```python
from build123d import *

# Parameters (mm, degrees)
EXTRUDE_1_DEPTH     = 30
SKETCH_2_R          = 10
CUT_EXTRUDE_1_DEPTH = 15
EXTRUDE_START       = 20
SKETCH_3_R          = 12.5
SKETCH_3_R_2        = 10
EXTRUDE_2_DEPTH     = 20


with BuildPart() as part:
    # 草图1 → 凸台-拉伸1 (new body)
    with BuildSketch(Plane(origin=(0, 0, 0), x_dir=(0, 0, -1), z_dir=(1, 0, 0))):
        Polygon((-1000, 30), (1000, 30), (1000, 0), (15, 0), (15, 15), (-15, 15), (-15, 0), (-1000, 0), align=None)
    extrude(amount=EXTRUDE_1_DEPTH)

    # 草图2 → 切除-拉伸1 (cut)
    with BuildSketch(Plane.XZ):
        with Locations(Location((15, 883.8834765, 0), (0, 0, 270))):
            Circle(SKETCH_2_R)
        with Locations(Location((15, -883.8834765, 0), (0, 0, 90))):
            Circle(SKETCH_2_R)
    extrude(amount=-CUT_EXTRUDE_1_DEPTH, mode=Mode.SUBTRACT)

    # 草图3 → 凸台-拉伸2 (add)
    # profile 1 of 2: a face of its own
    with BuildSketch(Plane.XZ.offset(EXTRUDE_START)):
        with Locations(Location((15, 883.8834765, 0), (0, 0, 90))):
            Circle(SKETCH_3_R)
        with Locations(Location((15, 883.8834765, 0), (0, 0, 270))):
            Circle(SKETCH_3_R_2, mode=Mode.SUBTRACT)
    # profile 2 of 2: a face of its own
    with BuildSketch(Plane.XZ.offset(EXTRUDE_START)):
        with Locations(Location((15, -883.8834765, 0), (0, 0, 90))):
            Circle(SKETCH_3_R)
        with Locations(Location((15, -883.8834765, 0), (0, 0, 90))):
            Circle(SKETCH_3_R_2, mode=Mode.SUBTRACT)
    extrude(amount=-EXTRUDE_2_DEPTH)


solid = part.part
```
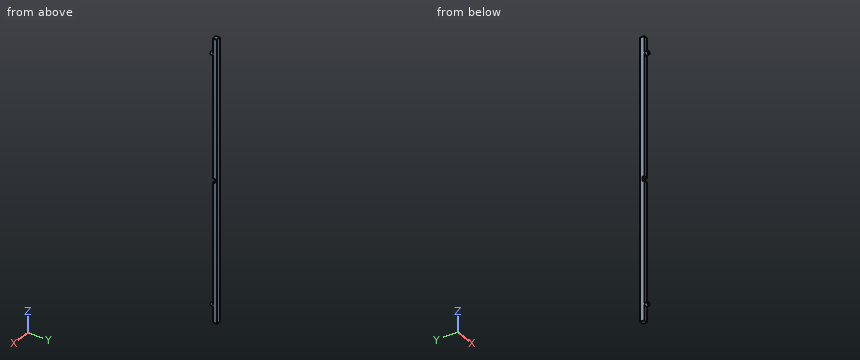
Input: part model. Units: mm. Frame: model coordinates. Give positions to 0.01 mm unless a question says otherwise; leave off trailing zeros. Order: outer loops, then holes, each group sorted by start corner. A loop starts at its lowest first (then second) coordinate and runs counter-clockwise, first axis right, second up.
1. Line query: probe 1 along Z at (x, y) = (17, 13); probe 2 along Z at (x, y) = (28.25, 6); probe 3 along Z at (x, y) = (11.75, -10.5). Output: solid intervals per line, ascending.
Computed:
probe 1: z = -1000 to -893.68, -874.09 to -15, 15 to 874.09, 893.68 to 1000
probe 2: z = -1000 to -15, 15 to 1000
probe 3: z = -895.95 to -893.34, -874.43 to -871.81, 871.81 to 874.43, 893.34 to 895.95
2. Cut plane A-A (y = -8.5). Return loops of the section in (x, z).
Computed:
outline: circle Ø25 at (15, -883.88); circle Ø25 at (15, 883.88); hole circle Ø20 at (15, -883.88); hole circle Ø20 at (15, 883.88)
3. Pin query (flat end, axial travel): pin 1 Ø3 at (x, y) = (10.5, -4.5) entering from +Z; pin 2 Ø18 at (x, z) = (15, 883.88) entering from -Y; pin 3 Ø2 at (x, y) = (10.5, -12) entering from -Z. Return the tip coordinate at first contact, or that it passes through.
Computed:
pin 1: stops at z = 896.02
pin 2: stops at y = 15
pin 3: stops at z = -895.88
4. Cut plane B-B (x = 15). Return loops of the section in (y, z).
Computed:
outline: (-20, -896.38) - (0, -896.38) - (0, -1000) - (30, -1000) - (30, 1000) - (0, 1000) - (0, 896.38) - (-20, 896.38) - (-20, 893.88) - (15, 893.88) - (15, 873.88) - (-20, 873.88) - (-20, 871.38) - (0, 871.38) - (0, 15) - (15, 15) - (15, -15) - (0, -15) - (0, -871.38) - (-20, -871.38) - (-20, -873.88) - (15, -873.88) - (15, -893.88) - (-20, -893.88) - close
5. Cut plane C-C (z = 256). Return loops of the section in (x, y).
Computed:
outline: (0, 0) - (30, 0) - (30, 30) - (0, 30) - close
